The drawing under review shows one solid part. Ordinate dimensions are in mm from its lowest x, y, z. A direction names the side the tool comes from. Round coordinates to 2 decimals unless told otherwise and drop trailing zeros. Write each loop counter-clockwise with the first axis right and the second up, starting at its lowest first coordinate (ties: lowest second). Pieces come first, ordered by that corner, then holes. Notation, with made-up numbers: M -9.75,-7.5 L -5.75,-7.5 A30 ccw -5.75,29.5 Z; hole C -37,3.25 d5. An arc over 180 degrees is marked long. Write item = value, one per line. Start each with the question number.
Item 1: To check wall thickness, follow line 1 along X through (y, z) = (13, 43.5); line 2 along Z through (x, y) = (17.75, 6.75); line 3 along Y through (x, z) = (21.5, 49.5) (1 decimal). State the ranges of each line that lie inside material, in increasing order.
Item 2: Tool access review of the marked faces 4, 5 and 6: name each direction out of +Z, -Z, +X, -X, +Y, -Y from which nothing blocks a thin tool from reaching the whole face with its end or side.
Item 3: Take a section at A-A, the plane x = 13. Give the boundary of the cut face in (y, z), plus the area to 3 significant figures.
Item 4: Take a section at B-B, the plane z = 35.5. Give the boundary of the cut face in (x, y).
Item 5: Take a section at D-D, the plane z = 56.5. Give the boundary of the cut face in (x, y), plus the area to 3 significant figures.
Item 6: For pin 1 Ø8 at (x, y) = (16.5, 13.5) entering from +Z; pin 2 Ø6 at (y, z) = (3.5, 38.5) entering from +X; pin 3 Ø5 at (y, z) = (10, 42.5) entering from +X; pin 4 Ø3 at (y, z) = (21.5, 39) entering from +X (1 decimal), all flat-tipped, find the tip position at first contact; note any pin that passes through.
Item 7: The part is to be moulded in two halves that separate along Z. For the marked faces 1, 2 and 3, say which applies: +Z half, -Z half, draft (parallel to the pull), parting line (faces both ways), or undercut.
Item 8: Take a section at C-C, the plane y = 9.25. Give the boundary of the cut face in (x, z), plus the area to 3 significant figures.
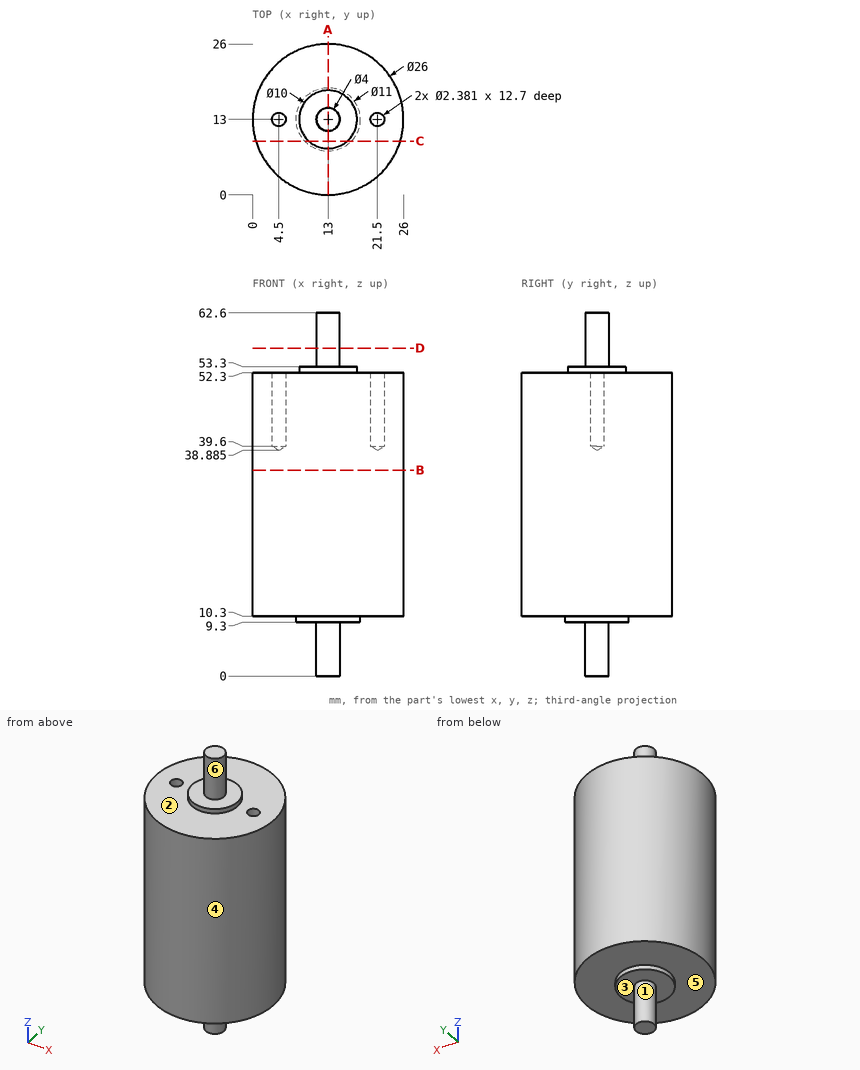
Response values:
q1.line_1 = 0 to 3.31, 5.69 to 20.31, 22.69 to 26
q1.line_2 = 10.3 to 52.3
q1.line_3 = 3.2 to 11.8, 14.2 to 22.8
q2.face_4 = +Z, -Z
q2.face_5 = -Z
q2.face_6 = +Z
q3.outline = M 0,10.3 L 7.5,10.3 L 7.5,9.3 L 11,9.3 L 11,0 L 15,0 L 15,9.3 L 18.5,9.3 L 18.5,10.3 L 26,10.3 L 26,52.3 L 18,52.3 L 18,53.3 L 15,53.3 L 15,62.6 L 11,62.6 L 11,53.3 L 8,53.3 L 8,52.3 L 0,52.3 Z
q3.area = 1,190 mm2
q4.outline = C 13,13 d26
q5.outline = C 13,13 d4
q5.area = 12.6 mm2
q6.pin_1 = 62.6
q6.pin_2 = 24.26
q6.pin_3 = 25.99
q6.pin_4 = 24
q7.face_1 = draft
q7.face_2 = +Z half
q7.face_3 = -Z half
q8.outline = M 0.55,10.3 L 8.98,10.3 L 8.98,9.3 L 17.02,9.3 L 17.02,10.3 L 25.45,10.3 L 25.45,52.3 L 16.31,52.3 L 16.31,53.3 L 9.69,53.3 L 9.69,52.3 L 0.55,52.3 Z
q8.area = 1,060 mm2
